Could you check a few things on this drawing? It's one solid part, dimensions in mm from its lowest x, y, z. Give positions to 0.01 mm unless a question says otherwise; leave off trailing zeros. Loops run counter-clockwise (first coordinate to the right, second up) from the corner with the lowest first, then second, coordinate; pieces in that order, holes last. Notation, with made-up numbers: (-37.5, -31.75) - (19.5, -31.75) arc R13 ccw to (19.5, -15.75) - close; hole circle Ø1 at (-17.5, -3.5). An arc over 180 degrees is marked (long way). Answer as a JSON object with one key per item and string values.
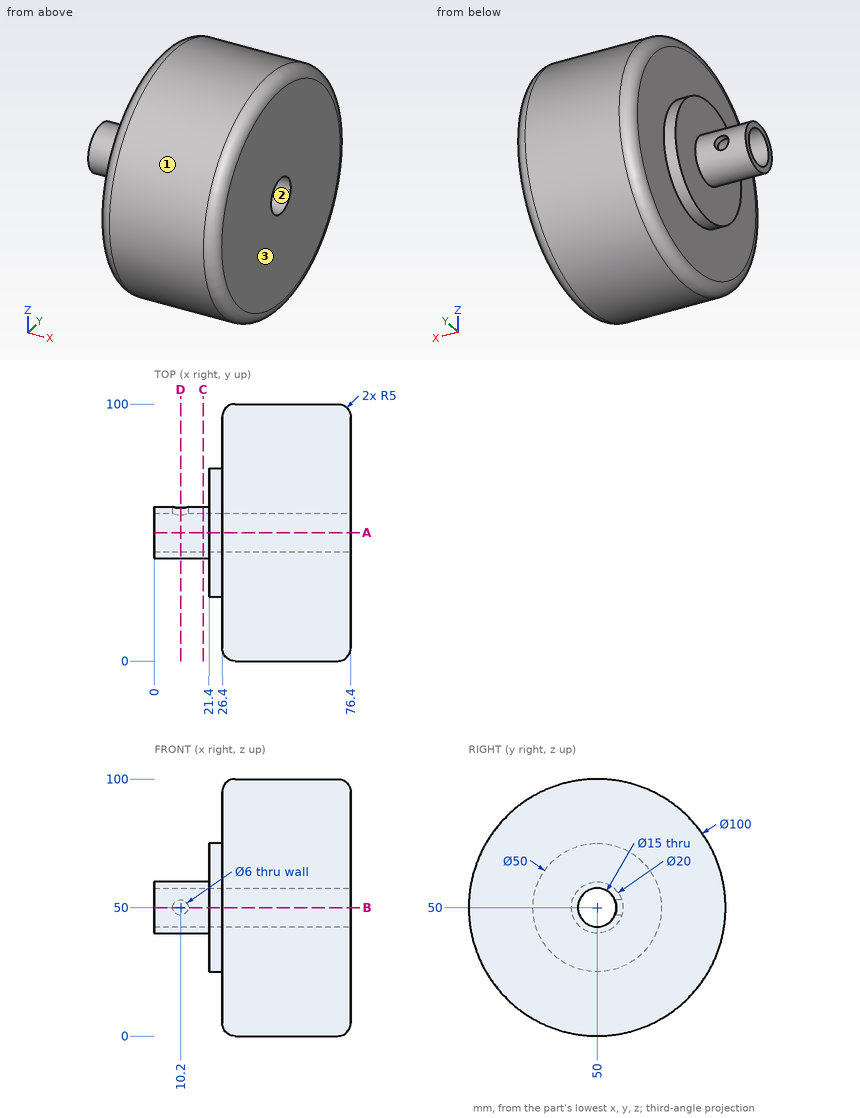
1) I'm going to push flat-ended pins straight in: P1, Ø2, axis at x = 65.5, z = 40.5, coming from the +Y side; P2, Ø8, axis at x = 10.2, z = 50, coming from the -Y side; P3, Ø2, axis at y = 22, z = 62.5, coming from the -X side. Where does each tip first touch, or does it pass through?
Check sheet entries:
{"P1": "y = 99.27", "P2": "y = 40", "P3": "x = 26.4"}
2) Imagine slicing it at D-D on x = 10.2. Write out the boundary of the cut face in (y, z).
Check sheet entries:
{"outline": "(56.87, 47) arc R7.5 cw (long way) to (56.87, 53) - (59.54, 53) arc R10 ccw (long way) to (59.54, 47) - close"}
3) If we mould it in two halves opening along Y, with no side actions, what happens to the marked faces 1, 2 and 3? For each: released by +Y, released by -Y, zero draft, split by the parting line, or undercut.
Check sheet entries:
{"face 1": "split by the parting line", "face 2": "undercut", "face 3": "zero draft"}
4) Imagine slicing it at C-C on x = 19. Write out the boundary of the cut face in (y, z), and give its area (3 significant figures).
Check sheet entries:
{"outline": "circle Ø20 at (50, 50); hole circle Ø15 at (50, 50)", "area": "137 mm2"}
5) I need wall thicknesses on L1, parallel to X at y = 58.75, z = 50; L2, parallel to X at y = 37, z = 79; L3, parallel to Z at x = 59, y = 51. Which ranges of each line are inside material? Lowest first, please.
Check sheet entries:
{"L1": "0 to 7.2, 13.2 to 76.4", "L2": "26.4 to 76.4", "L3": "0.01 to 42.57, 57.43 to 99.99"}
6) Imagine slicing it at A-A on y = 50. Write out the boundary of the cut face in (x, z).
Check sheet entries:
{"outline": "(0, 40) - (21.4, 40) - (21.4, 25) - (26.4, 25) - (26.4, 5) arc R5 ccw to (31.4, 0) - (71.4, 0) arc R5 ccw to (76.4, 5) - (76.4, 42.5) - (0, 42.5) - close; (0, 57.5) - (76.4, 57.5) - (76.4, 95) arc R5 ccw to (71.4, 100) - (31.4, 100) arc R5 ccw to (26.4, 95) - (26.4, 75) - (21.4, 75) - (21.4, 60) - (0, 60) - close"}
7) Imagine slicing it at B-B on z = 50. Write out the boundary of the cut face in (x, y), and give its area (3 significant figures).
Check sheet entries:
{"outline": "(0, 40) - (21.4, 40) - (21.4, 25) - (26.4, 25) - (26.4, 5) arc R5 ccw to (31.4, 0) - (71.4, 0) arc R5 ccw to (76.4, 5) - (76.4, 42.5) - (0, 42.5) - close; (0, 57.5) - (7.2, 57.5) - (7.2, 60) - (0, 60) - close; (13.2, 57.5) - (76.4, 57.5) - (76.4, 95) arc R5 ccw to (71.4, 100) - (31.4, 100) arc R5 ccw to (26.4, 95) - (26.4, 75) - (21.4, 75) - (21.4, 60) - (13.2, 60) - close", "area": "4,500 mm2"}
